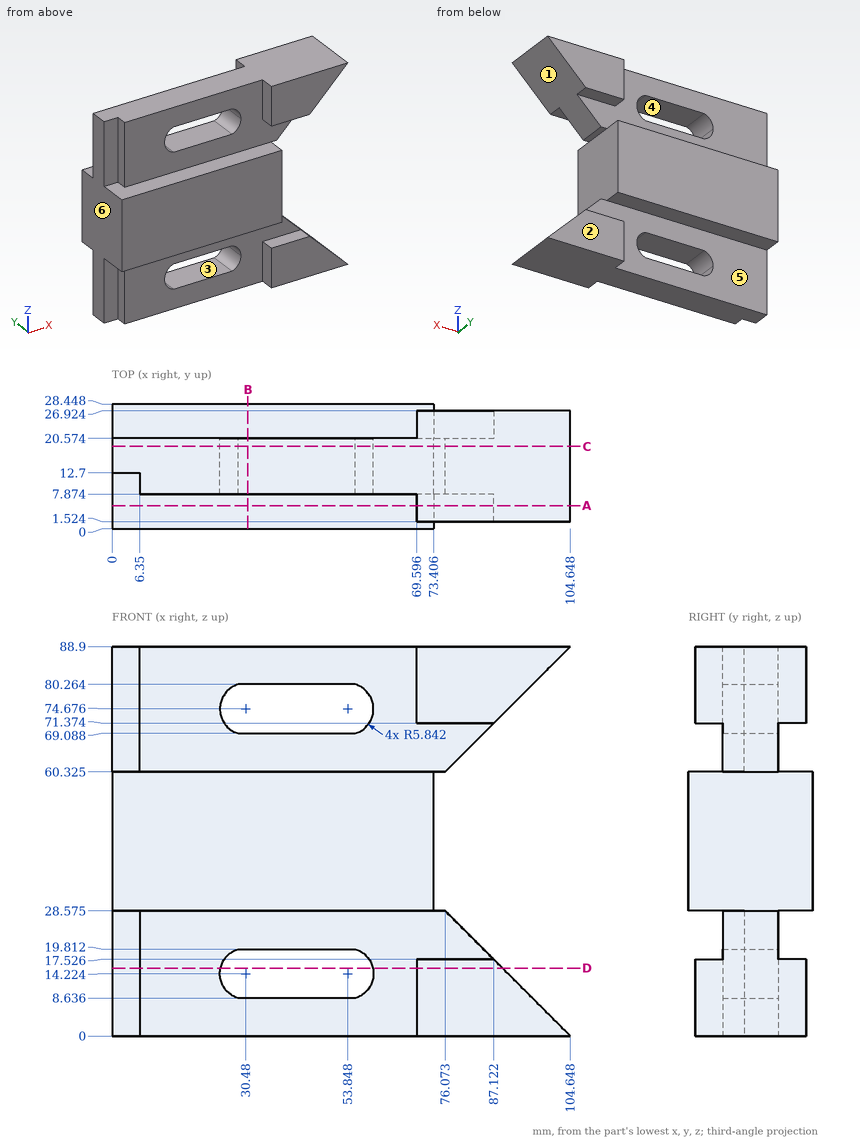
Study the drawing (mm; zero at the part's minimum x, y, z) and answer. A direction names the side the tool comes from. Coordinates: 2 decimals unless noted, no trailing zeros. Write each loop counter-clockwise with the first axis right and the second up, starting at its lowest first coordinate (ties: lowest second). Pieces come first, ordered by that corner, then holes. Notation, with made-up numbers: M 53,21.5 L 73,21.5 A25 ccw 73,57.5 Z; hole C 41.25,89 d3. An arc over 180 degrees is marked long. Write each question's results on one line, items separated by ' | '.
Item 1: The part is cut by section C-C on y = 18.75. Determine the outline of the cut face in (x, z) (3 decimals), and give its area (3 significant figures).
Answer below:
outline: M 0,0 L 104.648,0 L 76.073,28.575 L 73.406,28.575 L 73.406,60.325 L 76.073,60.325 L 104.648,88.9 L 0,88.9 Z; hole M 28.776,8.636 L 55.552,8.636 A5.842 ccw 55.552,19.812 L 28.776,19.812 A5.842 ccw Z; hole M 28.776,69.088 L 55.552,69.088 A5.842 ccw 55.552,80.264 L 28.776,80.264 A5.842 ccw Z | area: 6,760 mm2
Item 2: Consider probe 1 along Z at (x, y) = (52, 9.5); probe 2 along Z at (x, y) = (86, 3.25); probe 3 along Z at (x, y) = (15.5, 26.5) (3 decimals). Determine where each line is inside the solid, lowest interval first. Write a range as [from, to].
Answer below:
probe 1: [0, 8.64], [19.81, 69.09], [80.26, 88.9] | probe 2: [0, 17.53], [71.37, 88.9] | probe 3: [28.575, 60.325]
Item 3: The part is cut by section B-B on x = 31. Determine the outline of the cut face in (y, z) (3 decimals), and give its area (3 significant figures).
Answer below:
outline: M 0,28.575 L 7.874,28.575 L 7.874,19.812 L 20.574,19.812 L 20.574,28.575 L 28.448,28.575 L 28.448,60.325 L 20.574,60.325 L 20.574,69.088 L 7.874,69.088 L 7.874,60.325 L 0,60.325 Z; M 7.874,0 L 20.574,0 L 20.574,8.636 L 7.874,8.636 Z; M 7.874,80.264 L 20.574,80.264 L 20.574,88.9 L 7.874,88.9 Z | area: 1,350 mm2
Item 4: Given P1, Ø8, axis at y = 17, z = 25, coming from the +X side; P2, Ø8.5, axis at y = 9, z = 40.5, coming from the +X side; P3, Ø3, axis at y = 24, z = 10, coming from the -X side; P4, Ø4, axis at x = 56.5, z = 76.5, coming from the -Y side, each flat-ended and moving along its own axis, determine where each tip first touches the part or whether it passes through.
Answer below:
P1: x = 83.65 | P2: x = 73.41 | P3: x = 69.6 | P4: through
Item 5: For a pull along X with two mould halves and no side action, classify the marked faces 4, 5 and 6 as released by +X, released by -X, zero draft, split by the parting line, or undercut.
Answer below:
face 4: undercut | face 5: zero draft | face 6: released by -X
Item 6: The part is cut by section D-D on z = 15.5. Determine the outline of the cut face in (x, y), and give its area (3 significant figures).
Answer below:
outline: M 0,12.7 L 6.35,12.7 L 6.35,7.87 L 24.78,7.87 L 24.78,20.57 L 0,20.57 Z; M 59.55,7.87 L 69.6,7.87 L 69.6,1.52 L 89.15,1.52 L 89.15,26.92 L 69.6,26.92 L 69.6,20.57 L 59.55,20.57 Z | area: 908 mm2
Item 7: The part is cut by section A-A on y = 5.25. Determine the outline of the cut face in (x, z) (3 decimals).
Answer below:
outline: M 0,28.575 L 73.406,28.575 L 73.406,60.325 L 0,60.325 Z; M 69.596,0 L 104.648,0 L 87.122,17.526 L 69.596,17.526 Z; M 69.596,71.374 L 87.122,71.374 L 104.648,88.9 L 69.596,88.9 Z
Item 8: Which of the six approach directions +Z, -Z, +X, -X, +Y, -Y give full straight-line access (tool end or side, diameter ignored) to the marked faces 1, 2 and 3?
Answer below:
face 1: +X, +Y, -Y | face 2: -Z, +X, -X, +Y | face 3: +Y, -Y
